```python
from build123d import *

# Parameters (mm, degrees)
SKETCH004_W     = 22
SKETCH004_H     = 26
PAD003_DEPTH    = 2
SKETCH011_R     = 4.75
POCKET004_DEPTH = 2.001
SKETCH012_W     = 2
SKETCH012_H     = 15.2
PAD006_DEPTH    = 31.5
SKETCH014_R     = 1.3
POCKET006_DEPTH = 33.501
SKETCH015_W     = 18.2
SKETCH015_H     = 1.6
POCKET007_DEPTH = 6.85
FILLET_R        = 1


with BuildPart() as part:
    # Sketch004 → Pad003 (new body)
    with BuildSketch(Plane.XY):
        Rectangle(SKETCH004_W, SKETCH004_H)
    extrude(amount=PAD003_DEPTH)

    # Sketch011 (on Face6 of Pad003) → Pocket004 (cut, through all)
    with BuildSketch(Plane.XY.offset(2)):
        Circle(SKETCH011_R)
    extrude(amount=-POCKET004_DEPTH, mode=Mode.SUBTRACT)

    # Sketch012 (on Face4 of Pocket004) → Pad006 (join)
    with BuildSketch(Plane(origin=(0, 0, 0), x_dir=(1, 0, 0), z_dir=(0, 0, -1))):
        with Locations((-7.7, 0)):
            Rectangle(SKETCH012_W, SKETCH012_H)
        with Locations((7.7, 0)):
            Rectangle(SKETCH012_W, SKETCH012_H)
    extrude(amount=PAD006_DEPTH)

    # Sketch014 (on Face5 of Pad006) → Pocket006 (cut, through all)
    with BuildSketch(Plane.XY.offset(2)):
        with Locations((0, 10.5)):
            Circle(SKETCH014_R)
        with Locations((0, -10.5)):
            Circle(SKETCH014_R)
    extrude(amount=-POCKET006_DEPTH, mode=Mode.SUBTRACT)

    # Sketch015 (on Face18 of Pocket006) → Pocket007 (cut)
    with BuildSketch(Plane(origin=(0, 0, -31.5), x_dir=(1, 0, 0), z_dir=(0, 0, -1))):
        Rectangle(SKETCH015_W, SKETCH015_H)
    extrude(amount=-POCKET007_DEPTH, mode=Mode.SUBTRACT)

    # Fillet
    fillet_edges = [part.edges().sort_by_distance(p)[0] for p in [
        (11, -13, 1),
        (11, 13, 1),
        (-11, 13, 1),
        (-11, -13, 1),
    ]]
    fillet(fillet_edges, radius=FILLET_R)


with BuildPart() as part_1:
    # Body001 placement: moved
    add(part.part.moved(Location((0, 0, 48))))


solid = part_1.part
```
Input: part model. Units: mm. Frame: model coordinates. A direction names the side the tool comes from. Give positions to 0.01 mm unless a question says otherwise; leave off trailing zeros. Order: outer loops, then holes, each group sorted by start corner. A loop starts at its lowest first (then second) coordinate and runs counter-clockwise, first axis right, second up. Notation, with made-up numbers: (32.25, 15) -> (44.25, 15) arc R14 cw to (44.25, 41) -> close; hole circle Ø10 at (32, 40.25). An arc over 180 degrees is marked (long way). Write each question's results on one line, items separated by ' | '. Start each with the question number.
Item 1: Cut plane C-C on x = 0. Return the cut outline in (y, z).
Item 2: Line query: line 1 (Y direction, x = 0, z = 48.85); line 2 (X direction, y = -5.5, z = 18.5); line 3 (Z direction, x = 9.25, y = -1). Output: solid intervals per line, ascending.
Item 3: Cut plane D-D on y = 6. Return the cut outline in (x, z).
Item 4: Cut plane B-B on z = 31. Return the cut outline in (x, y).
Item 5: Contact query for flat-ended pins moving along their axis: P1, Ø2, axis at x = -7, z = 24.5, coming from the +Y side; P2, Ø1.6, axis at x = -8, z = 31.5, coming from the -Y side; P3, Ø0.5, axis at x = 8, y = 0.5, coming from the -Z side. Output: stop coordinate, or through.
Item 6: Mould query, pull axis Y, two halves, no side actions, for faces 4 (the flat face through (8, -7.6, 32)), 5 (the cylindrical face through (-10.715, 12.699, 49.014)), 6 (the flat face through (-8.7, 0, 32)), 7 (the flat face through (-8, 0.8, 20)). Classes: pulls with the +Y half, pulls with the -Y half, needs draft (parallel to the pull), parting line crosses it, or undercut.
Item 7: Set-up query: faces 1 (the flat face through (-8, 7.6, 32)), 2 (the flat face through (-6.7, 0, 32)), 3 (the flat face through (8, -0.8, 20)). Return all of +Z, -Z, +X, -X, +Y, -Y with unobstructed straight access to the full face (end or side cutting, diameter ignored); none if empty.
Item 8: Cut plane A-A on y = 10.5. Return the cut outline in (x, z), then the cut area to 3 significant figures.
Established:
1) outline: (-13, 48) -> (-11.8, 48) -> (-11.8, 50) -> (-13, 50) -> close; (-9.2, 48) -> (-4.75, 48) -> (-4.75, 50) -> (-9.2, 50) -> close; (4.75, 48) -> (9.2, 48) -> (9.2, 50) -> (4.75, 50) -> close; (11.8, 48) -> (13, 48) -> (13, 50) -> (11.8, 50) -> close
2) line 1: -13 to -11.8, -9.2 to -4.75, 4.75 to 9.2, 11.8 to 13 | line 2: -8.7 to -6.7, 6.7 to 8.7 | line 3: 48 to 50
3) outline: (-11, 48) -> (-8.7, 48) -> (-8.7, 16.5) -> (-6.7, 16.5) -> (-6.7, 48) -> (6.7, 48) -> (6.7, 16.5) -> (8.7, 16.5) -> (8.7, 48) -> (11, 48) -> (11, 50) -> (-11, 50) -> close
4) outline: (-8.7, -7.6) -> (-6.7, -7.6) -> (-6.7, 7.6) -> (-8.7, 7.6) -> close; (6.7, -7.6) -> (8.7, -7.6) -> (8.7, 7.6) -> (6.7, 7.6) -> close
5) P1: y = 7.6 | P2: y = -7.6 | P3: z = 23.35
6) face 4: pulls with the -Y half | face 5: pulls with the +Y half | face 6: needs draft | face 7: undercut
7) face 1: -Z, +X, -X, +Y | face 2: -Z, +Y, -Y | face 3: -Z, +X, -X
8) outline: (-11, 48) -> (-1.3, 48) -> (-1.3, 50) -> (-11, 50) -> close; (1.3, 48) -> (11, 48) -> (11, 50) -> (1.3, 50) -> close | area: 38.8 mm^2
